The listing builds one solid part. Answer for the finished solid, in the listing's coordinates (mm). A direction names the side the tool comes from. Coordinates: 2 decimals unless noted, no trailing zeros. Loops run counter-clockwise (first coordinate to the right, second up) from the corner with the lowest first, then second, coordinate; pieces in that order, holes last. Notation, with made-up numbers: M 53.25,-37 L 101.25,-37 A34 cw 101.25,-1 Z; hole C -40,-26 d3. An arc over 180 degrees is marked long. Answer in a Markdown table with one row per item. Add a question column.
from build123d import *

# Parameters (mm, degrees)
F0_W     = 15
F0_H     = 100
F1_DEPTH = 7.5
F2_R     = 7.5
F3_DEPTH = 17
F4_R     = 6.5
F5_DEPTH = 1
F6_R     = 7.5
F7_DEPTH = 2


with BuildPart() as f1:
    # F0 (on Top) → F1 (new body, symmetric)
    with BuildSketch(Plane.XY):
        with Locations((-7.5, 0)):
            Rectangle(F0_W, F0_H)
    extrude(amount=F1_DEPTH, both=True)

    # F2 (on face) → F3 (join)
    with BuildSketch(Plane.YZ):
        with Locations((42.5, 0)):
            Circle(F2_R)
    extrude(amount=F3_DEPTH)

    # F4 (on face) → F5 (join)
    with BuildSketch(Plane.YZ.offset(17)):
        with Locations((42.5, 0)):
            Circle(F4_R)
    extrude(amount=F5_DEPTH)

    # F6 (on face) → F7 (join)
    with BuildSketch(Plane.YZ.offset(18)):
        with Locations((42.5, 0)):
            Circle(F6_R)
    extrude(amount=F7_DEPTH)


solid = f1.part
(1) Straight lines are drawn through the part: line 1 (X direction, y = 35, z = 6.5); line 2 (Y direction, x = 11.5, z = -0.5); line 3 (Y direction, x = 6, z = -6.5). For each, find the intervals that lie inside material, in ascending order.
(2) The mould has two halves that part along X. Classify faces 1 (the face through (17.493, 36.006, 0.286)), 2 (the face through (-8, 1, 7.5)), 3 (the face through (-15, -1, 0)): released by +X, released by -X, zero draft, split by the parting line, or undercut.
(3) Each of these flat-tipped pins is pushed along its axis until it touches: pin 1 (4.5 mm diameter, centred on y = 1, z = 2, fed in from +X); pin 2 (1 mm diameter, centred on x = 7, z = 1.5, fed in from -Y); pin 3 (10 mm diameter, centred on x = 13.5, y = 35, fed in from -Z). Where does it stop, or does it pass through?
(4) For faces 4 (the face through (0, 48, 6)), 5 (the face through (18.986, 49.654, 2.253)), 6 (the face through (0, 48, -6)), determine the directions among +Z, -Z, +X, -X, +Y, -Y from which every point of the face is accessible in a straight line to the end or side of a thin tool.
(5) A cutting plane is placed at C-C (y = 22.5). Give the vertices of the cut face in (x, z).
(6) A cutting plane is placed at B-B (z = -5). Give the vertices of the cut face in (x, y).
(7) A cutting plane is placed at A-A (x = 13). Give the vertices of the cut face in (y, z).
Solved:
| question | item | result |
|---|---|---|
| 1 | line 1 | x = -15 to 0 |
| 1 | line 2 | y = 35.02 to 49.98 |
| 1 | line 3 | y = 38.76 to 46.24 |
| 2 | face 1 | undercut |
| 2 | face 2 | zero draft |
| 2 | face 3 | released by -X |
| 3 | pin 1 | stops at x = 0 |
| 3 | pin 2 | stops at y = 35.07 |
| 3 | pin 3 | stops at z = -7.07 |
| 4 | face 4 | +Z, +X, +Y |
| 4 | face 5 | +X |
| 4 | face 6 | -Z, +X, +Y |
| 5 | outline | M -15,-7.5 L 0,-7.5 L 0,7.5 L -15,7.5 Z |
| 6 | outline | M -15,-50 L 0,-50 L 0,36.91 L 17,36.91 L 17,38.35 L 18,38.35 L 18,36.91 L 20,36.91 L 20,48.09 L 18,48.09 L 18,46.65 L 17,46.65 L 17,48.09 L 0,48.09 L 0,50 L -15,50 Z |
| 7 | outline | C 42.5,0 d15 |
